```python
from build123d import *

# Parameters (mm, degrees)
SKETCH1_R                = 36.5
BOSS_EXTRUDE1_DEPTH      = 8
SKETCH2_R                = 27.5
BOSS_EXTRUDE2_DEPTH      = 14
SKETCH3_R                = 13
BOSS_EXTRUDE3_DEPTH      = 5
SKETCH4_R                = 7.5
CUT_EXTRUDE1_DEPTH       = 14
SKETCH6_R                = 7
BOSS_EXTRUDE4_DEPTH      = 10
BOSS_EXTRUDE4_DEPTH_BACK = 82
CUT_EXTRUDE2_DEPTH       = 12
SKETCH11_R               = 1.5
CUT_EXTRUDE4_DEPTH       = 28
FILLET1_R                = 2
SKETCH10_R               = 4.5
CUT_EXTRUDE5_DEPTH       = 93.0000001
SKETCH12_R               = 3.2
CUT_EXTRUDE6_DEPTH       = 14.0000001
SKETCH13_R               = 27.3
SKETCH13_R_2             = 25
CUT_EXTRUDE7_DEPTH       = 1.2
BOSS_EXTRUDE5_DEPTH      = 4
FILLET2_R                = 1
SKETCH15_R               = 1.5
CUT_EXTRUDE8_DEPTH       = 28
SKETCH16_W               = 25
SKETCH16_H               = 5.2
SKETCH17_R               = 4.5
CUT_EXTRUDE9_DEPTH       = 142
BOSS_EXTRUDE7_DEPTH      = 4
BOSS_EXTRUDE7_DEPTH_BACK = 16


with BuildPart() as part:
    # Sketch1 → Boss-Extrude1 (new body)
    with BuildSketch(Plane.XY):
        Circle(SKETCH1_R)
    extrude(amount=BOSS_EXTRUDE1_DEPTH)

    # Sketch2 → Boss-Extrude2 (add)
    with BuildSketch(Plane.XY.offset(8)):
        Circle(SKETCH2_R)
    extrude(amount=BOSS_EXTRUDE2_DEPTH)

    # Sketch3 → Boss-Extrude3 (add)
    with BuildSketch(Plane.XY.offset(22)):
        Circle(SKETCH3_R)
    extrude(amount=BOSS_EXTRUDE3_DEPTH)

    # Sketch4 → Cut-Extrude1 (cut)
    with BuildSketch(Plane.XY.offset(27)):
        Circle(SKETCH4_R)
    extrude(amount=-CUT_EXTRUDE1_DEPTH, mode=Mode.SUBTRACT)

    # Sketch6 → Boss-Extrude4 (add, two sides)
    with BuildSketch(Plane(origin=(36.5, 0, 0), x_dir=(0, 0, -1), z_dir=(1, 0, 0))) as boss_extrude4_sk:
        with Locations((-7, 12.5)):
            Circle(SKETCH6_R)
    extrude(amount=BOSS_EXTRUDE4_DEPTH)
    extrude(boss_extrude4_sk.sketch, amount=-BOSS_EXTRUDE4_DEPTH_BACK)

    # Sketch8 → Cut-Extrude2 (cut)
    with BuildSketch(Plane(origin=(0, 0, 0), x_dir=(-1, 0, 0), z_dir=(0, 0, -1))):
        with BuildLine():
            ThreePointArc((-17.653540721, 13.95), (0, -22.5), (17.653540721, 13.95))
            ThreePointArc((17.653540721, 13.95), (0, 18), (-17.653540721, 13.95))
        make_face()
    extrude(amount=-CUT_EXTRUDE2_DEPTH, mode=Mode.SUBTRACT)

    # Sketch11 → Cut-Extrude4 (cut, through all)
    with BuildSketch(Plane(origin=(0, 0, 0), x_dir=(-1, 0, 0), z_dir=(0, 0, -1))):
        with Locations((0, 31)):
            Circle(SKETCH11_R)
        with Locations((26.846787517, -15.5)):
            Circle(SKETCH11_R)
        with Locations((-26.846787517, -15.5)):
            Circle(SKETCH11_R)
    extrude(amount=-CUT_EXTRUDE4_DEPTH, mode=Mode.SUBTRACT)

    # Fillet1
    fillet1_edges = [part.edges().sort_by_distance(p)[0] for p in [
        (-27.5, 0, 22),
    ]]
    fillet(fillet1_edges, radius=FILLET1_R)

    # Sketch10 → Cut-Extrude5 (cut, through all)
    with BuildSketch(Plane(origin=(46.5, 0, 0), x_dir=(0, 0, -1), z_dir=(1, 0, 0))):
        with Locations((-7, 12.5)):
            Circle(SKETCH10_R)
    extrude(amount=-CUT_EXTRUDE5_DEPTH, mode=Mode.SUBTRACT)

    # Sketch12 → Cut-Extrude6 (cut, through all)
    with BuildSketch(Plane.XY.offset(13)):
        Circle(SKETCH12_R)
    extrude(amount=-CUT_EXTRUDE6_DEPTH, mode=Mode.SUBTRACT)

    # Sketch13 → Cut-Extrude7 (cut)
    with BuildSketch(Plane(origin=(0, 0, 0), x_dir=(-1, 0, 0), z_dir=(0, 0, -1))):
        Circle(SKETCH13_R)
        Circle(SKETCH13_R_2, mode=Mode.SUBTRACT)
    extrude(amount=-CUT_EXTRUDE7_DEPTH, mode=Mode.SUBTRACT)

    # Sketch14 → Boss-Extrude5 (add)
    with BuildSketch(Plane.XY.offset(8)):
        with BuildLine():
            Line((4.5, 31), (4.5, 27.129319933))
            ThreePointArc((4.5, 27.129319933), (0, 27.5), (-4.5, 27.129319933))
            Line((-4.5, 27.129319933), (-4.5, 31))
            ThreePointArc((-4.5, 31), (0, 35.5), (4.5, 31))
        make_face()
        with BuildLine():
            Line((29.096787517, -11.602885683), (25.744680249, -9.667545649))
            ThreePointArc((25.744680249, -9.667545649), (23.815698604, -13.75), (21.244680249, -17.461774283))
            Line((21.244680249, -17.461774283), (24.596787517, -19.397114317))
            ThreePointArc((24.596787517, -19.397114317), (30.743901834, -17.75), (29.096787517, -11.602885683))
        make_face()
        with BuildLine():
            Line((-24.596787517, -19.397114317), (-21.244680249, -17.461774283))
            ThreePointArc((-21.244680249, -17.461774283), (-23.815698604, -13.75), (-25.744680249, -9.667545649))
            Line((-25.744680249, -9.667545649), (-29.096787517, -11.602885683))
            ThreePointArc((-29.096787517, -11.602885683), (-30.743901834, -17.75), (-24.596787517, -19.397114317))
        make_face()
    extrude(amount=BOSS_EXTRUDE5_DEPTH)

    # Fillet2
    fillet2_edges = [part.edges().sort_by_distance(p)[0] for p in [
        (30.743901834, -17.75, 12),
        (27.420733883, -10.635215666, 12),
        (22.920733883, -18.4294443, 12),
        (-30.743901834, -17.75, 12),
        (-22.920733883, -18.4294443, 12),
        (-27.420733883, -10.635215666, 12),
        (0, 35.5, 12),
        (-4.5, 29.064659966, 12),
        (4.5, 29.064659966, 12),
    ]]
    fillet(fillet2_edges, radius=FILLET2_R)

    # Sketch15 → Cut-Extrude8 (cut, through all)
    with BuildSketch(Plane(origin=(0, 0, 0), x_dir=(-1, 0, 0), z_dir=(0, 0, -1))):
        with Locations((0, 31)):
            Circle(SKETCH15_R)
        with Locations((26.846787517, -15.5)):
            Circle(SKETCH15_R)
        with Locations((-26.846787517, -15.5)):
            Circle(SKETCH15_R)
    extrude(amount=-CUT_EXTRUDE8_DEPTH, mode=Mode.SUBTRACT)

    # Sketch16 → Revolve1 (revolve)
    with BuildSketch(Plane(origin=(0, 12.5, 0), x_dir=(1, 0, 0), z_dir=(0, 1, 0))):
        with Locations((-58, -9.6)):
            Rectangle(SKETCH16_W, SKETCH16_H)
        Polygon((-70.5, -12.2), (-70.5, -13), (-64.25, -13.65), (-64.25, -13), (-58, -13.65), (-58, -13), (-51.75, -13.65), (-51.75, -13), (-45.5, -13.65), (-45.5, -13), (-45.5, -12.2), align=None)
        Polygon((70.5, -13), (70.5, -7), (45.5, -7), (45.5, -13), (45.5, -13.65), (51.75, -13), (51.75, -13.65), (58, -13), (58, -13.65), (64.25, -13), (64.25, -13.65), align=None)
    revolve(axis=Axis((70.5, 12.5, 7), (-1, 0, 0)))

    # Sketch17 → Cut-Extrude9 (cut, through all)
    with BuildSketch(Plane(origin=(70.5, 0, 0), x_dir=(0, 0, -1), z_dir=(1, 0, 0))):
        with Locations((-7, 12.5)):
            Circle(SKETCH17_R)
    extrude(amount=-CUT_EXTRUDE9_DEPTH, mode=Mode.SUBTRACT)

    # Sketch18 → Boss-Extrude7 (add, two sides)
    with BuildSketch(Plane(origin=(0, 0, 4), x_dir=(-1, 0, 0), z_dir=(0, 0, -1))) as boss_extrude7_sk:
        with BuildLine():
            Line((-75, -32.5), (-36.282905966, -32.5))
            ThreePointArc((-36.282905966, -32.5), (-25.996296714, -27.748383535), (-21.244680249, -17.461774283))
            ThreePointArc((-21.244680249, -17.461774283), (0, -27.5), (21.244680249, -17.461774283))
            ThreePointArc((21.244680249, -17.461774283), (25.996296714, -27.748383535), (36.282905966, -32.5))
            Line((36.282905966, -32.5), (75, -32.5))
            Line((75, -32.5), (75, -40.5))
            Line((75, -40.5), (-75, -40.5))
            Line((-75, -40.5), (-75, -32.5))
        make_face()
    extrude(amount=BOSS_EXTRUDE7_DEPTH)
    extrude(boss_extrude7_sk.sketch, amount=-BOSS_EXTRUDE7_DEPTH_BACK)


solid = part.part
```
Build history of the part. All positions in model axes, mm. A direction names the side the tool comes from. Coordinates: 2 decimals unless noted, no trailing zeros. Write each loop counter-clockwise with the first axis right and the second up, starting at its lowest first coordinate (ties: lowest second). Pieces come first, ordered by that corner, then holes.
1. Drop flat-ended pins along their axis: pin 1 (14.5 mm diameter, centred on y = 14, z = 8.5, fed in from +X); pin 2 (6.5 mm diameter, centred on y = 11, z = 4.5, fed in from -X); pin 3 (1 mm diameter, centred on y = 3.5, z = 19, fed in from -X). Give the stop position or say it passes through.
Answer block:
pin 1: stops at x = 70.5
pin 2: stops at x = -70.5
pin 3: stops at x = -27.34
2. Band-saw the part on A-A, the plane x = -43. Give the cut face in (y, z).
Answer block:
outline: (-40.5, 0) - (-32.5, 0) - (-32.5, 20) - (-40.5, 20) - close; circle Ø14 at (12.5, 7); hole circle Ø9 at (12.5, 7)
3. Band-saw the part on B-B, the plane z = 16. Give the cut face in (x, y), and give its area (3 significant figures).
Answer block:
outline: (-75, -40.5) - (75, -40.5) - (75, -32.5) - (36.28, -32.5) arc R16.4 cw to (21.24, -17.46) arc R27.5 ccw (long way) to (-21.24, -17.46) arc R16.4 cw to (-36.28, -32.5) - (-75, -32.5) - close; hole circle Ø15 at (0, 0)
area: 3,850 mm2
4. Pull direction X, two halves, no side cores. Call faces 5 (the cylindrical face through (-0.1, 35.5, 9.5)), 6 (the flat face through (-1, -40.5, 10)), 7 (the flat face through (-27.397, -10.622, 9.479)), 8 (the cylindrical face through (28.345, -15.434, 5.916)): released by +X, released by -X, zero draft, split by the parting line, or undercut.
Answer block:
face 5: split by the parting line
face 6: zero draft
face 7: released by -X
face 8: undercut
5. 3-axis set-ups, long thin cutter, end or side, ignore diameter. For faces 1 (the conical face through (49.745, 8.722, 2.073)), 2 (the flat face through (4.5, 29, 9)), 3 (the cylindrical face through (30.69, -17.84, 9.48)), 4 (the cylindrical face through (36.175, 12.808, 13.993)): which of +Z, -Z, +X, -X, +Y, -Y reach the whole face in a straight line?
Answer block:
face 1: none
face 2: +Z, +X, +Y
face 3: +Z
face 4: +X
6. Drill centre lines: probe 1 along Y at (x, z) = (0, 3); probe 2 along Y at (x, z) = (0, 12.6); probe 3 along Y at (x, z) = (0, 22.75). Where is each one in solid material? Low to high.
Answer block:
probe 1: y = -40.5 to -22.5, 18 to 29.5, 32.5 to 36.5
probe 2: y = -40.5 to -3.2, 3.2 to 27.5
probe 3: y = -13 to -7.5, 7.5 to 13
7. Band-saw the part on D-D, the plane x = 0. Give the number of separate pieces and of enclosed holes in the cut face, and give its area (3 significant figures).
Answer block:
separate pieces: 3
enclosed holes: 0
area: 958 mm2
